```python
from build123d import *

# Parameters (mm, degrees)
SKETCH1_W           = 40
SKETCH1_H           = 160
SKETCH1_R           = 11
SKETCH1_R_2         = 10.5
BOSS_EXTRUDE1_DEPTH = 12
CUT_EXTRUDE3_REACH  = 85.331
SKETCH4_R           = 4
CUT_EXTRUDE4_REACH  = 163.691
SKETCH5_R           = 3


with BuildPart() as part:
    # Sketch1 → Boss-Extrude1 (new body)
    with BuildSketch(Plane(origin=(0, 0, 0), x_dir=(1, 0, 0), z_dir=(0, 1, 0))):
        Rectangle(SKETCH1_W, SKETCH1_H)
        with Locations(Location((0, 0, 0), (0, 0, 270))):
            Circle(SKETCH1_R, mode=Mode.SUBTRACT)
        with Locations(Location((0, 40, 0), (0, 0, 270))):
            Circle(SKETCH1_R_2, mode=Mode.SUBTRACT)
        with Locations(Location((0, -40, 0), (0, 0, 270))):
            Circle(SKETCH1_R_2, mode=Mode.SUBTRACT)
    extrude(amount=BOSS_EXTRUDE1_DEPTH)

    # Sketch4 → Cut-Extrude3 (cut, up to next)
    with BuildSketch(Plane(origin=(0, 12, 0), x_dir=(1, 0, 0), z_dir=(0, 1, 0)), mode=Mode.PRIVATE) as cut_extrude3_sk1:
        with Locations(Location((-10, 70, 0), (0, 0, 270))):
            Circle(SKETCH4_R)
    cut_extrude3_tool1 = extrude(cut_extrude3_sk1.sketch, amount=-CUT_EXTRUDE3_REACH, mode=Mode.PRIVATE) & part.part
    # Sketch4 → Cut-Extrude3 (cut, up to next)
    with BuildSketch(Plane(origin=(0, 12, 0), x_dir=(1, 0, 0), z_dir=(0, 1, 0)), mode=Mode.PRIVATE) as cut_extrude3_sk2:
        with Locations(Location((10, 70, 0), (0, 0, 270))):
            Circle(SKETCH4_R)
    cut_extrude3_tool2 = extrude(cut_extrude3_sk2.sketch, amount=-CUT_EXTRUDE3_REACH, mode=Mode.PRIVATE) & part.part
    cut_extrude3_1 = cut_extrude3_tool1.solids().sort_by_distance((-10, 12, -70))[0]
    add(cut_extrude3_1, mode=Mode.SUBTRACT)
    cut_extrude3_2 = cut_extrude3_tool2.solids().sort_by_distance((10, 12, -70))[0]
    add(cut_extrude3_2, mode=Mode.SUBTRACT)
    cut_extrude3 = cut_extrude3_1 + cut_extrude3_2  # Cut-Extrude3 as one shape, for the pattern or mirror that repeats it

    # Sketch5 → Cut-Extrude4 (cut, up to next)
    with BuildSketch(Plane(origin=(0, 0, -80), x_dir=(-1, 0, 0), z_dir=(0, 0, -1)), mode=Mode.PRIVATE) as cut_extrude4_sk1:
        with Locations((10, 6)):
            Circle(SKETCH5_R)
    cut_extrude4_tool1 = extrude(cut_extrude4_sk1.sketch, amount=-CUT_EXTRUDE4_REACH, mode=Mode.PRIVATE) & part.part
    # Sketch5 → Cut-Extrude4 (cut, up to next)
    with BuildSketch(Plane(origin=(0, 0, -80), x_dir=(-1, 0, 0), z_dir=(0, 0, -1)), mode=Mode.PRIVATE) as cut_extrude4_sk2:
        with Locations((-10, 6)):
            Circle(SKETCH5_R)
    cut_extrude4_tool2 = extrude(cut_extrude4_sk2.sketch, amount=-CUT_EXTRUDE4_REACH, mode=Mode.PRIVATE) & part.part
    cut_extrude4_1 = cut_extrude4_tool1.solids().sort_by_distance((-10, 6, -80))[0]
    add(cut_extrude4_1, mode=Mode.SUBTRACT)
    cut_extrude4_2 = cut_extrude4_tool2.solids().sort_by_distance((10, 6, -80))[0]
    add(cut_extrude4_2, mode=Mode.SUBTRACT)
    cut_extrude4 = cut_extrude4_1 + cut_extrude4_2  # Cut-Extrude4 as one shape, for the pattern or mirror that repeats it

    # Mirror1: Cut-Extrude3, Cut-Extrude4 across plane
    add(cut_extrude3.mirror(Plane.XY), mode=Mode.SUBTRACT)
    add(cut_extrude4.mirror(Plane.XY), mode=Mode.SUBTRACT)


solid = part.part
```
Geometry: final body of the model. Coordinates: model frame, mm. A direction names the side the tool comes from. Coordinates: 2 decimals unless noted, no trailing zeros. Order: outer loops, then holes, each group sorted by start corner. A loop starts at its lowest first (then second) coordinate and runs counter-clockwise, first axis right, second up.
Item 1: Section query C-C (x = 0). Output: boundary loops of the cut face in (y, z), then the cut area to 3 significant figures.
Answer:
outline: (0, -80) - (12, -80) - (12, -50.5) - (0, -50.5) - close; (0, -29.5) - (12, -29.5) - (12, -11) - (0, -11) - close; (0, 11) - (12, 11) - (12, 29.5) - (0, 29.5) - close; (0, 50.5) - (12, 50.5) - (12, 80) - (0, 80) - close
area: 1,150 mm2
Item 2: Section query A-A (z = -40). Output: boundary loops of the cut face in (x, y).
Answer:
outline: (-20, 0) - (-10.5, 0) - (-10.5, 12) - (-20, 12) - close; (10.5, 0) - (20, 0) - (20, 12) - (10.5, 12) - close
Item 3: Section query D-D (z = -70). Output: boundary loops of the cut face in (x, y).
Answer:
outline: (-20, 0) - (-14, 0) - (-14, 12) - (-20, 12) - close; (-6, 0) - (6, 0) - (6, 12) - (-6, 12) - close; (14, 0) - (20, 0) - (20, 12) - (14, 12) - close
Item 4: Material intervals for line 1 along X through (y, z) = (6, -76.5); line 2 along Z through (x, y) = (-0.5, 6.5); line 3 along X through (y, z) = (6.5, 70), sorted ascending.
Answer:
line 1: x = -20 to -13, -7 to 7, 13 to 20
line 2: z = -80 to -50.49, -29.51 to -10.99, 10.99 to 29.51, 50.49 to 80
line 3: x = -20 to -14, -6 to 6, 14 to 20
Item 5: Access query for faces 1 (the face through (0.46, 5.92, -50.49)), 2 (the face through (7.23, 4.85, -76.37)), 3 (the face through (7.23, 4.85, 76.37)). Directions: +Z, -Z, +X, -X, +Y, -Y. A direction counts if a zero-diameter tool reaches every point of the face in a straight line with its end or side. Return the directions, or none.
Answer:
face 1: +Y, -Y
face 2: -Z
face 3: +Z
Item 6: Section query B-B (y = 1.5). Output: boundary loops of the cut face in (x, z), then the cut area to 3 significant figures.
Answer:
outline: (-20, -80) - (20, -80) - (20, 80) - (-20, 80) - close; hole circle Ø8 at (-10, -70); hole circle Ø8 at (-10, 70); hole circle Ø22 at (0, 0); hole circle Ø21 at (0, -40); hole circle Ø21 at (0, 40); hole circle Ø8 at (10, -70); hole circle Ø8 at (10, 70)
area: 5,130 mm2
Item 7: Draft query along Z for faces 4 (the face through (0, 6, -80)), 5 (the face through (-14, 12, -1)), 6 (the face through (-8.799, 6.084, -66.185)). Return one class per face: released by +Z, released by -Z, zero draft, split by the parting line, or undercut.
Answer:
face 4: released by -Z
face 5: zero draft
face 6: undercut
Item 8: Contact query for flat-ended pins moving along their axis: P1, Ø3.5, axis at x = -10, y = 6, coming from the -Z side; P2, Ø5.5, axis at x = 10, y = 6, coming from the -Z side. Output: stop coordinate, or through.
Answer:
P1: stops at z = -66.4
P2: stops at z = -67.1
